Build history of the part. All positions in model axes, mm. Face numbers are marked on the shaded views. A direction names the side the tool comes from. Round coordinates to 2 decimals unless told otherwise and drop trailing zeros. Write each loop counter-clockwise with the first axis right and the second up, starting at its lowest first coordinate (ties: lowest second). Pieces come first, ordered by that corner, then holes.
1) Wall check: probe 1 along Z at (x, y) = (7, -1); probe 2 along Y at (x, z) = (14, -9.5); probe 3 along Z at (x, y) = (7.75, -0.7). Give the ranges that are in metal, low to high.
2) Saw through at D-D (x = 7.75). Write the cut outline in (y, z), plus the area to 3 significant figures.
3) Saw through at B-B (x = 0). Write the cut outline in (y, z), plus the area to 3 significant figures.
4) Saw through at A-A (z = 0). Write the cut outline in (x, y).
5) Which spindle directions (+Z, -Z, +X, -X, +Y, -Y) get a long thin tool onto all of the face, cutting with end or side? Do the marked faces 1, 2 and 3. Say none if no direction does.
6) Saw through at C-C (y = -53). Write the cut outline in (x, z), plus the area to 3 significant figures.
7) Flat gauge pins, fed straight in: pin 1 (3 mm diameter, centred on x = 0.5, y = 4, fed in from +Z); pin 2 (4 mm diameter, centred on x = 15.5, z = 0, fed in from +Y); pin 3 (5 mm diameter, centred on y = 3, z = 5, fed in from +X); pin 4 (12 mm diameter, centred on x = 13.5, z = -14.5, fed in from -Y). Where does each tip first touch, or does it go through?
Autodesk Fusion 360 part; units mm, degrees
sketch "Sketch1" plane through (0, 0, 0) normal (0, 1, 0) x (1, 0, 0)
  circle A0 centre (0, 0) radius 18.5
  dimension "d1" = 37
extrude "Extrude1" add sketch "Sketch1" against normal blind 25
sketch "Sketch2" plane through (0, -25, 0) normal (0, -1, 0) x (1, 0, 0)
  circle A0 centre (0, 0) radius 18.5
  circle A1 centre (0, 0) radius 16
  dimension "d4" = 32
extrude "Extrude2" add sketch "Sketch2" along normal blind 41 contours A1
sketch "Sketch3" plane through (0, 0, 0) normal (0, 1, 0) x (-1, 0, 0)
  circle A0 centre (0, 0) radius 18.5
  line L0 (0, 0) -> (0, 7)
  circle A1 centre (0, 7) radius 6
  dimension "d7" = 7
  dimension "d8" = 12
extrude "Extrude3" add sketch "Sketch3" along normal blind 7 contours A1
sketch "Sketch4" plane through (0, 7, 0) normal (0, 1, 0) x (-1, 0, 0)
  circle A0 centre (0, 7) radius 6
  circle A1 centre (0, 7) radius 3
  dimension "d11" = 6
extrude "Extrude4" add sketch "Sketch4" along normal blind 15.5 contours A1
sketch "Sketch5" plane through (0, 0, 0) normal (0, 1, 0) x (-1, 0, 0)
  circle A0 centre (0, 7) radius 6
  circle A1 centre (0, 0) radius 18.5
  line L0 (0, 0) -> (15.5, 0)
  circle A2 centre (15.5, 0) radius 1.5
  circle A3 centre (7.75, 13.4234) radius 1.5
  circle A4 centre (-7.75, 13.4234) radius 1.5
  circle A5 centre (-15.5, 0) radius 1.5
  circle A6 centre (-7.75, -13.4234) radius 1.5
  circle A7 centre (7.75, -13.4234) radius 1.5
  dimension "d14" = 3
  dimension "d15" = 15.5
  dimension "d17" = 360
extrude "Extrude5" cut sketch "Sketch5" against normal blind 3.5 contours A2 | A3 | A4 | A5 | A6 | A7
sketch "Sketch6" plane through (0, 22.5, 0) normal (0, 1, 0) x (-1, 0, 0)
  circle A0 centre (0, 7) radius 3
  circle A1 centre (0, 7) radius 3
  line L0 (0, 7) -> (0, 9.5)
  line L1 (0, 9.5) -> (-1.6583, 9.5)
  line L2 (0, 9.5) -> (1.6583, 9.5)
extrude "Extrude6" cut sketch "Sketch6" against normal blind 12 contours A0 A1 L1 L2 picked at (-0.1459, 9.8226)
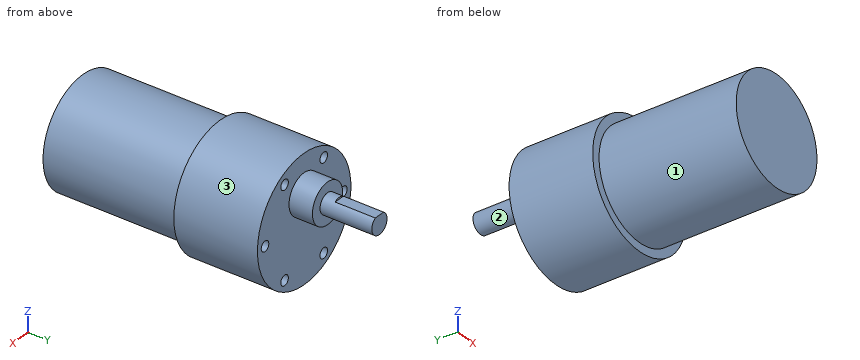
Evaluation:
1. probe 1: z = -17.12 to -14.72, -12.12 to 12.12, 14.72 to 17.12
1. probe 2: y = -25 to 0
1. probe 3: z = -16.8 to -14.92, -11.92 to 11.92, 14.92 to 16.8
2. outline: (-66, -14) - (-25, -14) - (-25, -16.8) - (0, -16.8) - (0, -14.92) - (-3.5, -14.92) - (-3.5, -11.92) - (0, -11.92) - (0, 11.92) - (-3.5, 11.92) - (-3.5, 14.92) - (0, 14.92) - (0, 16.8) - (-25, 16.8) - (-25, 14) - (-66, 14) - close
2. area: 1,970 mm2
3. outline: (-66, -16) - (-25, -16) - (-25, -18.5) - (0, -18.5) - (0, 1) - (7, 1) - (7, 4) - (22.5, 4) - (22.5, 9.5) - (10.5, 9.5) - (10.5, 10) - (7, 10) - (7, 13) - (0, 13) - (0, 18.5) - (-25, 18.5) - (-25, 16) - (-66, 16) - close
3. area: 2,410 mm2
4. outline: (-18.5, -25) - (-16, -25) - (-16, -66) - (16, -66) - (16, -25) - (18.5, -25) - (18.5, 0) - (17, 0) - (17, -3.5) - (14, -3.5) - (14, 0) - (-14, 0) - (-14, -3.5) - (-17, -3.5) - (-17, 0) - (-18.5, 0) - close
5. face 1: -Y
5. face 2: +Y
5. face 3: +Y, -Y
6. outline: circle Ø32 at (0, 0)
6. area: 804 mm2
7. pin 1: stops at z = 13
7. pin 2: stops at y = 0
7. pin 3: stops at x = 6
7. pin 4: stops at y = -66
